Read the model definition and answer for the solid it produces. Units are mm, in the model's axes. Coordinates: 2 decimals unless noted, no trailing zeros. Order: outer loops, then holes, each group sorted by start corner. A loop starts at its lowest first (then second) coordinate and runs counter-clockwise, first axis right, second up. Notation, with made-up numbers: M -27.5,-28.5 L 9.5,-28.5 A8 cw 9.5,-13.5 Z; hole C -26,21 d10. An arc over 180 degrees is marked long. Write each question's results on one line, items separated by ' | '.
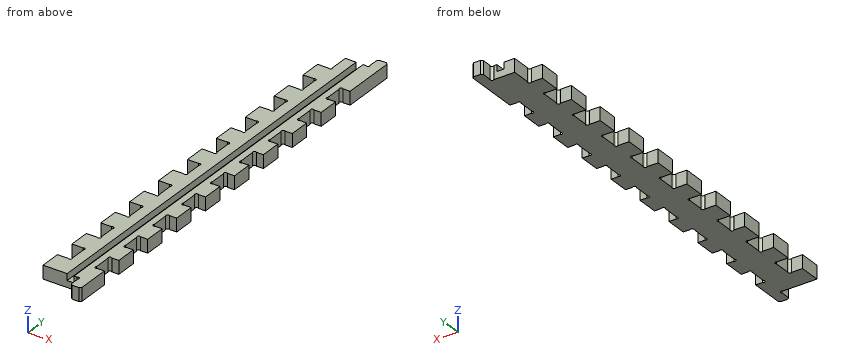
```python
from build123d import *

# Parameters (mm, degrees)
BOSS_EXTRUDE1_DEPTH = 6.35
CUT_EXTRUDE1_DEPTH  = 3.175
CHAMFER1_SIZE       = 0.79375
SKETCH5_W           = 3.302
SKETCH5_H           = 3.175
CUT_EXTRUDE4_DEPTH  = 208.663320883


# Read off the part's stored shape, not the designer's step: Boss-Extrude1
with BuildPart() as part:
    # Boss-Extrude1 outline → Boss-Extrude1 (new body)
    with BuildSketch(Plane.XY):
        with BuildLine():
            Line((22.436796564, 150), (19.069200519, 150))
            ThreePointArc((19.069200519, 150), (17.946668504, 150), (17.946668504, 151.122532015))
            Line((17.946668504, 151.122532015), (17.946668504, 158.877467985))
            ThreePointArc((17.946668504, 158.877467985), (17.946668504, 160), (19.069200519, 160))
            Line((19.069200519, 160), (22.436796564, 160))
            Line((22.436796564, 160), (22.436796564, 170))
            Line((22.436796564, 170), (19.069200519, 170))
            ThreePointArc((19.069200519, 170), (17.946668504, 170), (17.946668504, 171.122532015))
            Line((17.946668504, 171.122532015), (17.946668504, 178.877467985))
            ThreePointArc((17.946668504, 178.877467985), (17.946668504, 180), (19.069200519, 180))
            Line((19.069200519, 180), (22.436796564, 180))
            Line((22.436796564, 180), (22.436796564, 206.35))
            Line((22.436796564, 206.35), (17.436796564, 206.35))
            Line((17.436796564, 206.35), (17.436796564, 201.122532015))
            ThreePointArc((17.436796564, 201.122532015), (17.436796564, 200), (16.314264549, 200))
            Line((16.314264549, 200), (6.35, 200))
            Line((6.35, 200), (6.35, 191.122532015))
            ThreePointArc((6.35, 191.122532015), (6.35, 190), (5.227467985, 190))
            Line((5.227467985, 190), (0, 190))
            Line((0, 190), (0, 180))
            Line((0, 180), (5.227467985, 180))
            ThreePointArc((5.227467985, 180), (6.35, 180), (6.35, 178.877467985))
            Line((6.35, 178.877467985), (6.35, 171.122532015))
            ThreePointArc((6.35, 171.122532015), (6.35, 170), (5.227467985, 170))
            Line((5.227467985, 170), (0, 170))
            Line((0, 170), (0, 160))
            Line((0, 160), (5.227467985, 160))
            ThreePointArc((5.227467985, 160), (6.35, 160), (6.35, 158.877467985))
            Line((6.35, 158.877467985), (6.35, 151.122532015))
            ThreePointArc((6.35, 151.122532015), (6.35, 150), (5.227467985, 150))
            Line((5.227467985, 150), (0, 150))
            Line((0, 150), (0, 140))
            Line((0, 140), (5.227467985, 140))
            ThreePointArc((5.227467985, 140), (6.35, 140), (6.35, 138.877467985))
            Line((6.35, 138.877467985), (6.35, 131.122532015))
            ThreePointArc((6.35, 131.122532015), (6.35, 130), (5.227467985, 130))
            Line((5.227467985, 130), (0, 130))
            Line((0, 130), (0, 120))
            Line((0, 120), (5.227467985, 120))
            ThreePointArc((5.227467985, 120), (6.35, 120), (6.35, 118.877467985))
            Line((6.35, 118.877467985), (6.35, 111.122532015))
            ThreePointArc((6.35, 111.122532015), (6.35, 110), (5.227467985, 110))
            Line((5.227467985, 110), (0, 110))
            Line((0, 110), (0, 100))
            Line((0, 100), (5.227467985, 100))
            ThreePointArc((5.227467985, 100), (6.35, 100), (6.35, 98.877467985))
            Line((6.35, 98.877467985), (6.35, 91.122532015))
            ThreePointArc((6.35, 91.122532015), (6.35, 90), (5.227467985, 90))
            Line((5.227467985, 90), (0, 90))
            Line((0, 90), (0, 80))
            Line((0, 80), (5.227467985, 80))
            ThreePointArc((5.227467985, 80), (6.35, 80), (6.35, 78.877467985))
            Line((6.35, 78.877467985), (6.35, 71.122532015))
            ThreePointArc((6.35, 71.122532015), (6.35, 70), (5.227467985, 70))
            Line((5.227467985, 70), (0, 70))
            Line((0, 70), (0, 60))
            Line((0, 60), (5.227467985, 60))
            ThreePointArc((5.227467985, 60), (6.35, 60), (6.35, 58.877467985))
            Line((6.35, 58.877467985), (6.35, 51.122532015))
            ThreePointArc((6.35, 51.122532015), (6.35, 50), (5.227467985, 50))
            Line((5.227467985, 50), (0, 50))
            Line((0, 50), (0, 40))
            Line((0, 40), (5.227467985, 40))
            ThreePointArc((5.227467985, 40), (6.35, 40), (6.35, 38.877467985))
            Line((6.35, 38.877467985), (6.35, 31.122532015))
            ThreePointArc((6.35, 31.122532015), (6.35, 30), (5.227467985, 30))
            Line((5.227467985, 30), (0, 30))
            Line((0, 30), (0, 20))
            Line((0, 20), (5.227467985, 20))
            ThreePointArc((5.227467985, 20), (6.35, 20), (6.35, 18.877467985))
            Line((6.35, 18.877467985), (6.35, 11.122532015))
            ThreePointArc((6.35, 11.122532015), (6.35, 10), (5.227467985, 10))
            Line((5.227467985, 10), (0, 10))
            Line((0, 10), (0, 0))
            Line((0, 0), (16.314264549, 0))
            ThreePointArc((16.314264549, 0), (17.436796564, 0), (17.436796564, -1.122532015))
            Line((17.436796564, -1.122532015), (17.436796564, -6.35))
            Line((17.436796564, -6.35), (22.436796564, -6.35))
            Line((22.436796564, -6.35), (22.436796564, 10))
            Line((22.436796564, 10), (19.069200519, 10))
            ThreePointArc((19.069200519, 10), (17.946668504, 10), (17.946668504, 11.122532015))
            Line((17.946668504, 11.122532015), (17.946668504, 18.877467985))
            ThreePointArc((17.946668504, 18.877467985), (17.946668504, 20), (19.069200519, 20))
            Line((19.069200519, 20), (22.436796564, 20))
            Line((22.436796564, 20), (22.436796564, 30))
            Line((22.436796564, 30), (19.069200519, 30))
            ThreePointArc((19.069200519, 30), (17.946668504, 30), (17.946668504, 31.122532015))
            Line((17.946668504, 31.122532015), (17.946668504, 38.877467985))
            ThreePointArc((17.946668504, 38.877467985), (17.946668504, 40), (19.069200519, 40))
            Line((19.069200519, 40), (22.436796564, 40))
            Line((22.436796564, 40), (22.436796564, 50))
            Line((22.436796564, 50), (19.069200519, 50))
            ThreePointArc((19.069200519, 50), (17.946668504, 50), (17.946668504, 51.122532015))
            Line((17.946668504, 51.122532015), (17.946668504, 58.877467985))
            ThreePointArc((17.946668504, 58.877467985), (17.946668504, 60), (19.069200519, 60))
            Line((19.069200519, 60), (22.436796564, 60))
            Line((22.436796564, 60), (22.436796564, 70))
            Line((22.436796564, 70), (19.069200519, 70))
            ThreePointArc((19.069200519, 70), (17.946668504, 70), (17.946668504, 71.122532015))
            Line((17.946668504, 71.122532015), (17.946668504, 78.877467985))
            ThreePointArc((17.946668504, 78.877467985), (17.946668504, 80), (19.069200519, 80))
            Line((19.069200519, 80), (22.436796564, 80))
            Line((22.436796564, 80), (22.436796564, 90))
            Line((22.436796564, 90), (19.069200519, 90))
            ThreePointArc((19.069200519, 90), (17.946668504, 90), (17.946668504, 91.122532015))
            Line((17.946668504, 91.122532015), (17.946668504, 98.877467985))
            ThreePointArc((17.946668504, 98.877467985), (17.946668504, 100), (19.069200519, 100))
            Line((19.069200519, 100), (22.436796564, 100))
            Line((22.436796564, 100), (22.436796564, 110))
            Line((22.436796564, 110), (19.069200519, 110))
            ThreePointArc((19.069200519, 110), (17.946668504, 110), (17.946668504, 111.122532015))
            Line((17.946668504, 111.122532015), (17.946668504, 118.877467985))
            ThreePointArc((17.946668504, 118.877467985), (17.946668504, 120), (19.069200519, 120))
            Line((19.069200519, 120), (22.436796564, 120))
            Line((22.436796564, 120), (22.436796564, 130))
            Line((22.436796564, 130), (19.069200519, 130))
            ThreePointArc((19.069200519, 130), (17.946668504, 130), (17.946668504, 131.122532015))
            Line((17.946668504, 131.122532015), (17.946668504, 138.877467985))
            ThreePointArc((17.946668504, 138.877467985), (17.946668504, 140), (19.069200519, 140))
            Line((19.069200519, 140), (22.436796564, 140))
            Line((22.436796564, 140), (22.436796564, 150))
        make_face()
    extrude(amount=BOSS_EXTRUDE1_DEPTH)

    # Sketch2 → Cut-Extrude1 (cut)
    with BuildSketch(Plane.XY.offset(6.35)):
        Polygon((14.771668504, -1.25), (11.596668504, -1.25), (11.596668504, 200), (11.596668504, 201.5875), (14.771668504, 201.5875), (14.771668504, 0), align=None)
    extrude(amount=-CUT_EXTRUDE1_DEPTH, mode=Mode.SUBTRACT)

    # Chamfer1
    chamfer1_edges = [part.edges().sort_by_distance(p)[0] for p in [
        (22.436796564, -6.35, 3.175),
        (17.436796564, -6.35, 3.175),
        (17.436796564, 206.35, 3.175),
        (22.436796564, 206.35, 3.175),
    ]]
    chamfer(chamfer1_edges, length=CHAMFER1_SIZE)

    # Sketch5 → Cut-Extrude4 (cut, through all)
    with BuildSketch(Plane(origin=(0, 200, 0), x_dir=(1, 0, 0), z_dir=(0, 1, 0))):
        with Locations((13.184168504, -4.7625)):
            Rectangle(SKETCH5_W, SKETCH5_H)
    extrude(amount=-CUT_EXTRUDE4_DEPTH, mode=Mode.SUBTRACT)


solid = part.part
```
(1) Given pin 1 (1.6 mm diameter, centred on y = 77, z = 5, fed in from +X); pin 2 (3 mm diameter, centred on x = 3.5, y = 75.5, fed in from +Z); pin 3 (3.5 mm diameter, centred on y = 203.5, z = 4.5, fed in from -X); pin 4 (1.6 mm diameter, centred on x = 3.5, z = 4.5, fed in from -Y), each flat-ended and moving along its own axis, determine where each tip first touches the part or whether it passes through.
Conclusion:
pin 1: x = 17.95 | pin 2: through | pin 3: x = 17.44 | pin 4: y = 0
(2) The part is cut by section B-B, the plane y = 76. Write down the section's boundary in (x, z) (3 decimals), then the cut area to 3 significant figures.
Conclusion:
outline: M 6.35,0 L 17.947,0 L 17.947,6.35 L 14.835,6.35 L 14.835,3.175 L 11.533,3.175 L 11.533,6.35 L 6.35,6.35 Z | area: 63.2 mm²
(3) The part is cut by section A-A, the plane y = 164. Write down the section's boundary in (x, z) (3 decimals).
Conclusion:
outline: M 0,0 L 22.437,0 L 22.437,6.35 L 14.835,6.35 L 14.835,3.175 L 11.533,3.175 L 11.533,6.35 L 0,6.35 Z
(4) Straight lines are drawn through the part: line 1 (X direction, y = 123.5, z = 4.75); line 2 (X direction, y = 196.5, z = 5); line 3 (Z direction, x = 13.25, y = 139) (3 decimals). For each, find the intervals that lie inside material, in ascending order.
Conclusion:
line 1: 0 to 11.53, 14.84 to 22.44 | line 2: 6.35 to 11.53, 14.84 to 22.44 | line 3: 0 to 3.175
